Model file for the job. Use its own axes, mm. A direction names the side the tool comes from. Round coordinates to 2 decimals unless told otherwise and drop trailing zeros. Order: outer loops, then holes, each group sorted by start corner. A loop starts at its lowest first (then second) coordinate and runs counter-clockwise, first axis right, second up. Notation, with made-up numbers: (4.5, 27) -> (25.5, 27) arc R17 ccw to (25.5, 45) -> close; hole circle Ø3 at (36.5, 34.25). An arc over 180 degrees is marked (long way). Use CSV: the item, a comma, the result in double quotes.
```python
from build123d import *

# Parameters (mm, degrees)
EXTRUDE_1_DEPTH     = 394
SKETCH_2_R          = 1.5
SKETCH_2_W          = 44
SKETCH_2_H          = 22
CUT_EXTRUDE_1_DEPTH = 411.987848396
FILLET_1_R          = 3


with BuildPart() as part:
    # 草图1 → 凸台-拉伸1 (new body)
    with BuildSketch(Plane.XY):
        Polygon((0, 0), (0, 116), (1.5, 116), (1.5, 0.401923789), (14.799038106, -22.632685902), (13.5, -23.382685902), align=None)
    extrude(amount=EXTRUDE_1_DEPTH)

    # 草图2 → 切除-拉伸1 (cut, through all)
    with BuildSketch(Plane.ZY):
        with Locations((385, 24)):
            Circle(SKETCH_2_R)
        with Locations((385, 102)):
            Circle(SKETCH_2_R)
        with Locations((9, 102)):
            Circle(SKETCH_2_R)
        with Locations((9, 24)):
            Circle(SKETCH_2_R)
        with Locations((156, 35)):
            Rectangle(SKETCH_2_W, SKETCH_2_H)
        with Locations((238, 35)):
            Rectangle(SKETCH_2_W, SKETCH_2_H)
        with Locations((302, 35)):
            Rectangle(SKETCH_2_W, SKETCH_2_H)
        with Locations((92, 35)):
            Rectangle(SKETCH_2_W, SKETCH_2_H)
    extrude(amount=-CUT_EXTRUDE_1_DEPTH, mode=Mode.SUBTRACT)

    # 圆角1
    fillet_1_edges = [part.edges().sort_by_distance(p)[0] for p in [
        (0.75, 24, 216),
        (0.75, 46, 216),
        (0.75, 46, 260),
        (0.75, 24, 260),
        (0.75, 24, 280),
        (0.75, 46, 280),
        (0.75, 46, 324),
        (0.75, 24, 324),
        (0.75, 46, 178),
        (0.75, 24, 178),
        (0.75, 24, 134),
        (0.75, 46, 134),
        (0.75, 46, 70),
        (0.75, 46, 114),
        (0.75, 24, 114),
        (0.75, 24, 70),
    ]]
    fillet(fillet_1_edges, radius=FILLET_1_R)


solid = part.part
```
Q1. Pin check, flat tips, straight feed: pin 1 (1.6 mm diameter, centred on x = 1, z = 159, fed in from -Y); pin 2 (6 mm diameter, centred on x = 6.5, z = 184, fed in from +Y); pin 3 (1 mm diameter, centred on x = 3.5, z = 220, fed in from +Y); pin 4 (1.2 mm diameter, centred on x = 0.5, y = 32, fed in from -Z). Stop position of each tip, or through.
From the geometry:
pin 1,"stops at y = -3.12"
pin 2,"stops at y = -3.06"
pin 3,"stops at y = -2.2"
pin 4,"stops at z = 0"
Q2. Cut at B-B (z = 55.5). Give the cut face in (x, y), plus the area to 3 significant figures.
From the geometry:
outline,"(0, 0) -> (13.5, -23.38) -> (14.8, -22.63) -> (1.5, 0.4) -> (1.5, 116) -> (0, 116) -> close"
area,"214 mm²"
Q3. Cut at C-C (x = 5). Give the cut face in (y, z), plus the area to 3 significant figures.
From the geometry:
outline,"(-8.66, 0) -> (-5.66, 0) -> (-5.66, 394) -> (-8.66, 394) -> close"
area,"1,180 mm²"
Q4. Which spindle directions (+Z, -Z, +X, -X, +Y, -Y) get a long thin tool onto all of the face, cutting with end or side? Do faces 1 (the flat face through (0, 57, 194)), 2 (the flat face through (1.5, 59, 194)). Say none if no direction does.
From the geometry:
face 1,"+Z, -Z, -X, +Y, -Y"
face 2,"+Z, -Z, +X, +Y"
Q5. Probe line 1 along Z through (x, y) = (0.75, 102); line 2 along Y through (x, z) = (0.75, 9); line 3 along X through (y, z) = (109, 303). List the from-to ranges inside material, lowest first.
From the geometry:
line 1,"z = 0 to 7.5, 10.5 to 383.5, 386.5 to 394"
line 2,"y = -1.3 to 22.5, 25.5 to 100.5, 103.5 to 116"
line 3,"x = 0 to 1.5"
Q6. Cut at A-A (z = 141.5). Give the cut face in (x, y).
From the geometry:
outline,"(0, 0) -> (13.5, -23.38) -> (14.8, -22.63) -> (1.5, 0.4) -> (1.5, 24) -> (0, 24) -> close; (0, 46) -> (1.5, 46) -> (1.5, 116) -> (0, 116) -> close"
